For this review, take the finished solid that the model builds, in its own axes (mm). Face numbers are marked on the shaded views. A direction names the side the tool comes from. Give positions to 0.01 mm unless a question says otherwise; leave off trailing zeros. Loops run counter-clockwise (first coordinate to the right, second up) from the corner with the lowest first, then second, coordinate; pieces in that order, holes last.
```python
from build123d import *

# Parameters (mm, degrees)
F1_DEPTH = 25.4
F2_R     = 6.350053
F3_DEPTH = 25.4
F4_R     = 7.19822
F5_DEPTH = 25.4
F6_R     = 5.510191
F7_DEPTH = 25.4


with BuildPart() as f1:
    # F0 (on Front) → F1 (new body)
    with BuildSketch(Plane.XZ):
        Polygon((0, 12.7), (0, 0), (76.2, 0), (76.2, 12.911667), (44.45, 12.911667), (44.45, 44.45), (19.05, 44.45), (19.05, 12.7), align=None)
    extrude(amount=F1_DEPTH)

    # F2 (on face) → F3 (cut)
    with BuildSketch(Plane.YZ.offset(44.45)):
        with BuildLine():
            ThreePointArc((-25.4, 37.126943), (-12.537074, 44.028554), (0, 36.55133))
            Line((0, 36.55133), (0, 44.45))
            Line((0, 44.45), (-25.4, 44.45))
            Line((-25.4, 44.45), (-25.4, 37.126943))
        make_face()
        with Locations((-12.663453, 31.75)):
            Circle(F2_R)
    extrude(amount=-F3_DEPTH, mode=Mode.SUBTRACT)

    # F4 (on face) → F5 (cut)
    with BuildSketch(Plane.XY.offset(12.911667)):
        with Locations((57.15, -12.7)):
            Circle(F4_R)
        with BuildLine():
            ThreePointArc((63.5, 0), (71.379619, -12.7), (63.5, -25.4))
            Line((63.5, -25.4), (76.2, -25.4))
            Line((76.2, -25.4), (76.2, 0))
            Line((76.2, 0), (63.5, 0))
        make_face()
    extrude(amount=-F5_DEPTH, mode=Mode.SUBTRACT)

    # F6 (on face) → F7 (cut)
    with BuildSketch(Plane.XY.offset(12.7)):
        with BuildLine():
            ThreePointArc((6.35, -25.4), (0.149355, -12.7), (6.35, 0))
            Line((6.35, 0), (0, 0))
            Line((0, 0), (0, -25.4))
            Line((0, -25.4), (6.35, -25.4))
        make_face()
        with Locations((12.7, -12.7)):
            Circle(F6_R)
    extrude(amount=-F7_DEPTH, mode=Mode.SUBTRACT)


solid = f1.part
```
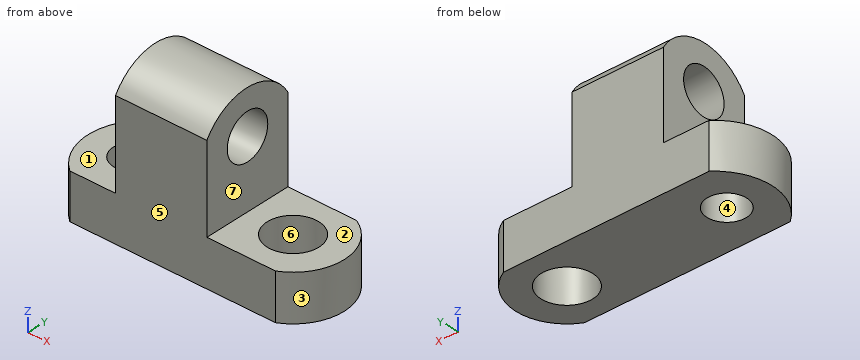
Item 1: Clearance check with flat-ended pins moving along their axes: pin 1 Ø1 at (x, y) = (37, -15.5) entering from +Z; pin 2 Ø3 at (y, z) = (-19.5, 19) entering from -X; pin 3 Ø5 at (y, z) = (-23, 10) entering from -X. State where each tip first meets the part, or that it passes through.
Answer:
pin 1: stops at z = 43.88
pin 2: stops at x = 19.05
pin 3: stops at x = 2.16
Item 2: Tool access review of the marked faces 1, 2 and 3: name each direction out of +Z, -Z, +X, -X, +Y, -Y from which nothing blocks a thin tool from reaching the whole face with its end or side.
Answer:
face 1: +Z, -X, +Y, -Y
face 2: +Z, +X, +Y, -Y
face 3: +Z, -Z, +X
Item 3: Take a section at C-C on y = -9.5. Give the boundary of the cut face in (x, z).
Answer:
outline: (0.47, 0) - (8.21, 0) - (8.21, 12.7) - (0.47, 12.7) - close; (17.19, 0) - (50.7, 0) - (50.7, 12.91) - (44.45, 12.91) - (44.45, 26.24) - (19.05, 26.24) - (19.05, 12.7) - (17.19, 12.7) - close; (19.05, 37.26) - (44.45, 37.26) - (44.45, 43.64) - (19.05, 43.64) - close; (63.6, 0) - (71.01, 0) - (71.01, 12.91) - (63.6, 12.91) - close
Item 4: For L1, parallel to X at y = -12, z = 8; L2, parallel to Z at x = 9.5, y = -4.25; L3, parallel to Y at x = 12.7, z = 7.75, list the stretches that pass through material, from the lowest coordinate up.
Answer:
L1: x = 0.16 to 7.23, 18.17 to 49.99, 64.31 to 71.36
L2: z = 0 to 12.7
L3: y = -25.4 to -18.21, -7.19 to 0
Item 5: Take a section at B-B on x = 12.7. Give the boundary of the cut face in (y, z), and give its area (3 significant figures).
Answer:
outline: (-25.4, 0) - (-18.21, 0) - (-18.21, 12.7) - (-25.4, 12.7) - close; (-7.19, 0) - (0, 0) - (0, 12.7) - (-7.19, 12.7) - close
area: 183 mm2
Item 6: Take a section at A-A on z = 31.75. Give the boundary of the cut face in (x, y), and give its area (3 significant figures).
Answer:
outline: (19.05, -25.4) - (44.45, -25.4) - (44.45, -19.01) - (19.05, -19.01) - close; (19.05, -6.31) - (44.45, -6.31) - (44.45, 0) - (19.05, 0) - close
area: 323 mm2
Item 7: Take a section at D-D on x = 40. Give the boundary of the cut face in (y, z), and give its area (3 significant figures).
Answer:
outline: (-25.4, 0) - (0, 0) - (0, 36.55) arc R14.82 ccw to (-25.4, 37.13) - close; hole circle Ø12.7 at (-12.66, 31.75)
area: 938 mm2
Item 8: The part is to be moulded in two halves that separate along Y. For the marked faces 4, 5, 6 and 7, say which applies: released by +Y, released by -Y, zero draft, split by the parting line, or undercut.
Answer:
face 4: undercut
face 5: released by -Y
face 6: undercut
face 7: zero draft
